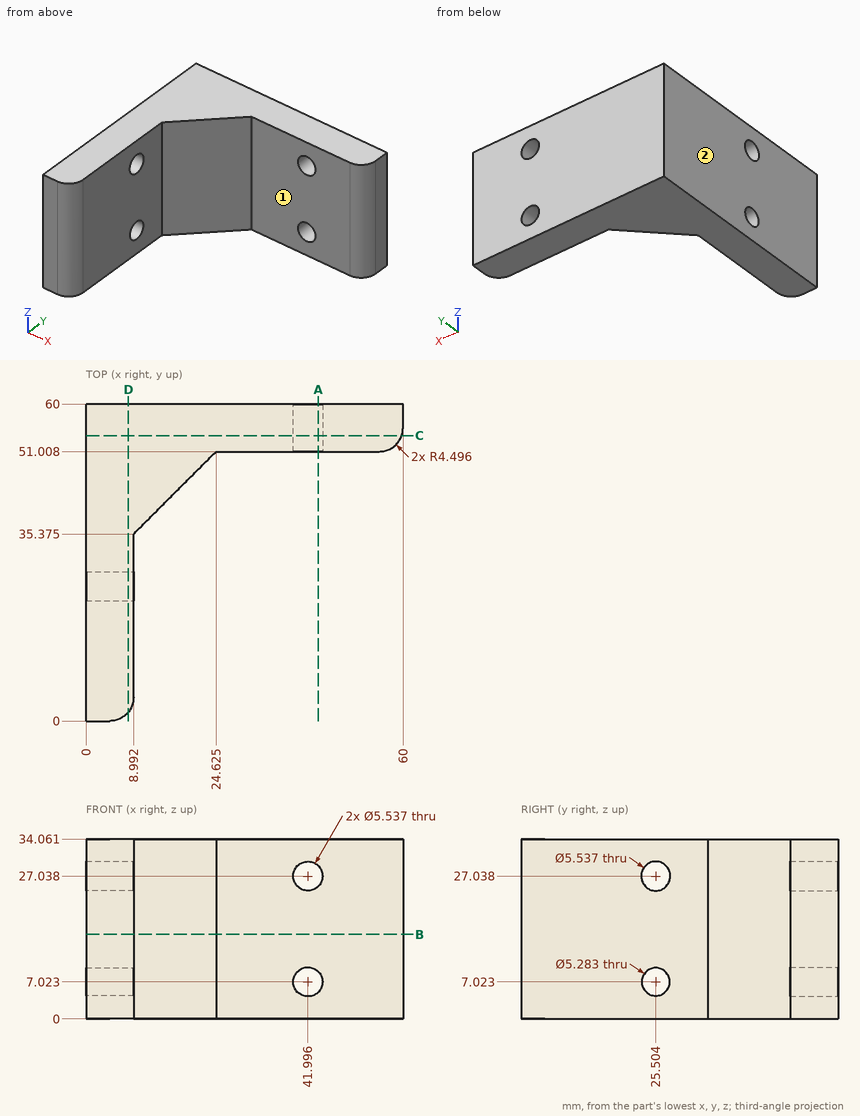
The figure shows three views and two pictorial views of one solid part (mm, origin at its lowest corner). Answer the questions. A direction names the side the tool comes from. Give positions to 0.01 mm unless a question says otherwise; leave off trailing zeros. Order: outer loops, then holes, each group sorted by start corner. A loop starts at its lowest first (then second) coordinate and runs counter-clockwise, first axis right, second up. Notation, with made-up numbers: (46.5, -30) -> (51.5, -30) arc R25 cw to (51.5, -9) -> close; hole circle Ø5 at (-6.75, 12.5). An arc over 180 degrees is marked (long way). One line per item, written item: value.
1) Find section A-A, the plane x = 44. Determine the outline of the cut face in (y, z).
Reported:
outline: (51.01, 0) -> (60, 0) -> (60, 5.11) -> (51.01, 5.11) -> close; (51.01, 8.93) -> (60, 8.93) -> (60, 25.13) -> (51.01, 25.13) -> close; (51.01, 28.95) -> (60, 28.95) -> (60, 34.06) -> (51.01, 34.06) -> close
2) Find section C-C, the plane y = 54. Determine the outline of the cut face in (x, z) (1 decimal), plus the area to 3 significant figures.
Reported:
outline: (0, 0) -> (59.7, 0) -> (59.7, 34.1) -> (0, 34.1) -> close; hole circle Ø5.5 at (42, 7); hole circle Ø5.5 at (42, 27)
area: 1,990 mm^2
3) A tool of negligible diameter and unlimited length cuts with its end or side. For the marked faces 1 and 2, from which of +Z, -Z, +X, -X, +Y, -Y can it reach the whole face along a straight path? Write none if from no direction.
Reported:
face 1: +Z, -Z, +X, -Y
face 2: +Z, -Z, -X, +Y, -Y
4) Find section B-B, the plane z = 16. Determine the outline of the cut face in (x, y) (1 decimal).
Reported:
outline: (0, 0) -> (4.5, 0) arc R4.5 ccw to (9, 4.5) -> (9, 35.4) -> (24.6, 51) -> (55.5, 51) arc R4.5 ccw to (60, 55.5) -> (60, 60) -> (0, 60) -> close
5) Find section D-D, the plane x = 8. Determine the outline of the cut face in (y, z) (1 decimal), plus the area to 3 significant figures.
Reported:
outline: (1.7, 0) -> (60, 0) -> (60, 34.1) -> (1.7, 34.1) -> close; hole circle Ø5.5 at (25.5, 27); hole circle Ø5.3 at (25.5, 7)
area: 1,940 mm^2
6) Flat-ended cylindrical pins translate along their axes: P1, Ø8, axis at y = 16.5, z = 13, coming from the -X side; P2, Ø10, axis at x = 20, z = 27, coming from the -Y side; P3, Ø1, axis at y = 49, z = 20.5, coming from the +X side; P4, Ø4.5, axis at x = 42, z = 27.04, coming from the +Y side. Find the tip coordinate at first contact, or state that the pin passes through.
Reported:
P1: stops at x = 0
P2: stops at y = 41.38
P3: stops at x = 23.12
P4: passes through
7) Find the intervals of material crossed by line 1 (Y direction, x = 28.5, z = 32.5); line 2 (X direction, y = 35, z = 6.5); line 3 (Y direction, x = 7, z = 8.5) (1 decimal), in increasing order.
Reported:
line 1: y = 51.01 to 60
line 2: x = 0 to 8.99
line 3: y = 0.8 to 23.3, 27.7 to 60
